For this review, use the dimensioned drawing (mm, ordinates from the lowest corner) and the shaded views. Round coordinates to 2 decimals unless told otherwise and drop trailing zeros. Order: outer loops, then holes, each group sorted by start corner. A loop starts at its lowest first (then second) coordinate and runs counter-clockwise, first axis right, second up. Notation, with made-up numbers: (-17.75, 55) - (0.25, 55) arc R9 cw to (0.25, 59) - close; hole circle Ø7 at (2.25, 21). An arc over 180 degrees is marked (long way). Write item = value, one per line.
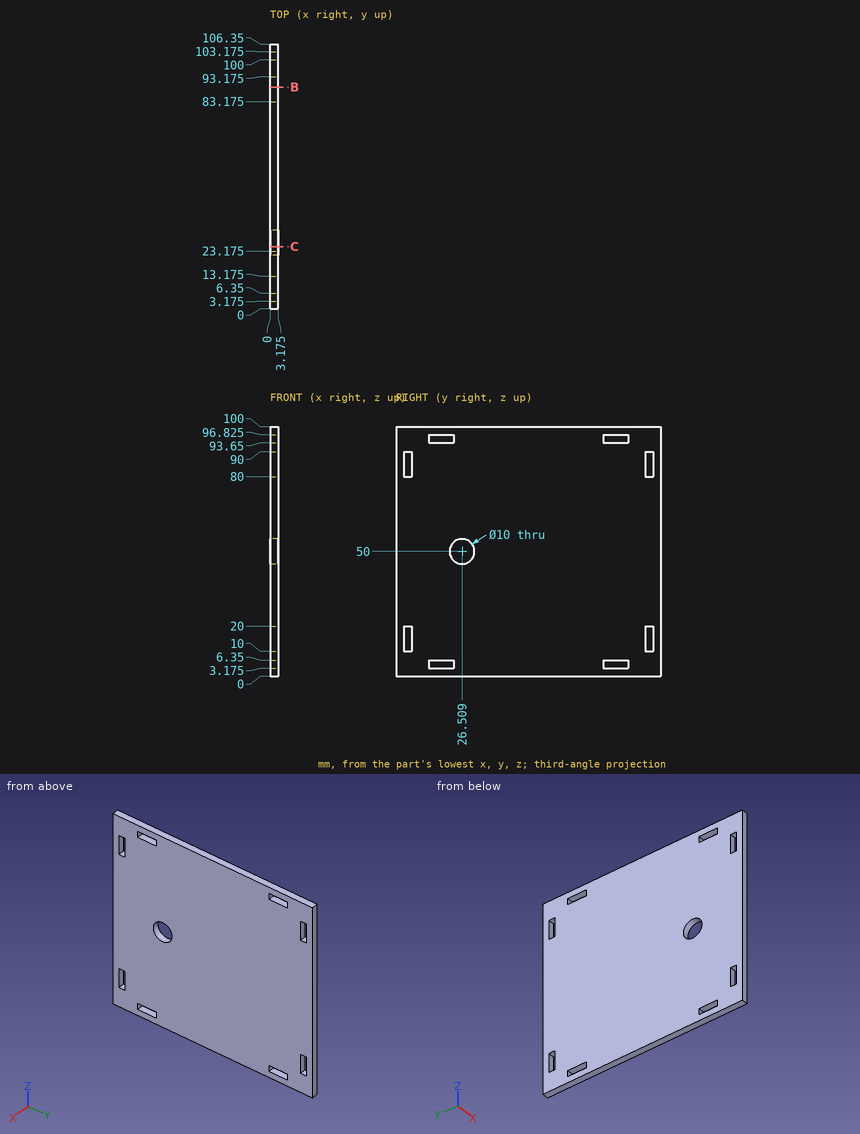
1) To check wall thickness, follow L1, parallel to Y at x = 2.25, z = 50; L2, parallel to Y at x = 0.25, z = 47. State the ranges of each line that lie inside material, in increasing order. Write a range as from..to.
Findings:
L1 = 0..21.51, 31.51..106.35
L2 = 0..22.51, 30.51..106.35
2) We need section B-B on y = 89. Give the number of separate pieces and of enclosed holes in the cut face, and give its area (3 significant figures).
Findings:
separate_pieces = 3
enclosed_holes = 0
area = 297 mm^2
3) We need section C-C on y = 25. Write out the cut boundary in (x, z) (1 decimal), and give its area (3 significant figures).
Findings:
outline = (0, 0) - (3.2, 0) - (3.2, 45.2) - (0, 45.2) - close; (0, 54.8) - (3.2, 54.8) - (3.2, 100) - (0, 100) - close
area = 287 mm^2
